from build123d import *

# Parameters (mm, degrees)
F1_DEPTH = 6.35
F3_DEPTH = 3.175


with BuildPart() as f1:
    # F0 (on Top) → F1 (new body)
    with BuildSketch(Plane.XY):
        with BuildLine():
            Line((44.45, 50.8), (-44.45, 50.8))
            ThreePointArc((-44.45, 50.8), (-48.940128, 48.940128), (-50.8, 44.45))
            Line((-50.8, 44.45), (-50.8, -44.45))
            ThreePointArc((-50.8, -44.45), (-48.940128, -48.940128), (-44.45, -50.8))
            Line((-44.45, -50.8), (44.45, -50.8))
            ThreePointArc((44.45, -50.8), (48.940128, -48.940128), (50.8, -44.45))
            Line((50.8, -44.45), (50.8, 44.45))
            ThreePointArc((50.8, 44.45), (48.940128, 48.940128), (44.45, 50.8))
        make_face()
    extrude(amount=F1_DEPTH)

    # F2 (on face) → F3 (cut)
    with BuildSketch(Plane.XY.offset(6.35)):
        Polygon((-2.234112, -19.045804), (-29.552355, -19.045804), (-29.552355, -21.484036), (-5.271634, -21.484036), (-5.271634, -27.478021), (-32.396957, -27.478021), (-32.396957, -31.338554), (-5.271634, -31.338554), (-5.271634, -37.027761), (-37.070233, -37.027761), (-37.070233, -24.125453), (-15.844628, 34.422915), (0, 34.422915), (15.844628, 34.422915), (37.070233, -24.125453), (37.070233, -37.027761), (5.271634, -37.027761), (5.271634, -31.338554), (32.396957, -31.338554), (32.396957, -27.478021), (5.271634, -27.478021), (5.271634, -21.484036), (29.552355, -21.484036), (29.552355, -19.045804), (2.234112, -19.045804), (2.234112, -40.488526), (41.246254, -40.488526), (41.246254, -24.237618), (17.566774, 37.974838), (0, 37.974838), (-17.566774, 37.974838), (-41.246254, -24.237618), (-41.246254, -40.488526), (-2.234112, -40.488526), align=None)
        with BuildLine():
            ThreePointArc((-9.515172, 23.211), (-17.458093, 10.48697), (-14.43387, -4.204695))
            ThreePointArc((-14.43387, -4.204695), (-2.520981, -10.7353), (10.401524, -6.543092))
            ThreePointArc((10.401524, -6.543092), (-4.451794, -8.46966), (-15.078945, 2.084788))
            ThreePointArc((-15.078945, 2.084788), (-12.326603, 15.929623), (0, 22.807829))
            ThreePointArc((0, 22.807829), (6.601318, 22.159177), (12.001306, 18.307129))
            ThreePointArc((12.001306, 18.307129), (14.956093, 7.863629), (9.017832, -1.221222))
            ThreePointArc((9.017832, -1.221222), (0.186781, -1.812212), (-5.294772, 5.136839))
            ThreePointArc((-5.294772, 5.136839), (-4.342036, 9.759367), (-0.376268, 12.318302))
            ThreePointArc((-0.376268, 12.318302), (-0.337375, 12.329109), (-0.301231, 12.347085))
            ThreePointArc((-0.301231, 12.347085), (3.122709, 12.777502), (5.674904, 10.454805))
            ThreePointArc((5.674904, 10.454805), (5.988125, 7.475454), (4.115821, 5.136839))
            ThreePointArc((4.115821, 5.136839), (1.688211, 5.89567), (0.35678, 8.062788))
            ThreePointArc((0.35678, 8.062788), (-0.732404, 6.827583), (-0.7692, 5.181162))
            ThreePointArc((-0.7692, 5.181162), (-0.749973, 5.13983), (-0.722364, 5.103558))
            ThreePointArc((-0.722364, 5.103558), (1.991164, 3.466413), (5.160289, 3.455573))
            ThreePointArc((5.160289, 3.455573), (8.487959, 7.340866), (7.337417, 12.325357))
            ThreePointArc((7.337417, 12.325357), (2.944683, 15.261206), (-2.33871, 15.228196))
            ThreePointArc((-2.33871, 15.228196), (-7.7104, 9.043988), (-7.555628, 0.854024))
            ThreePointArc((-7.555628, 0.854024), (-6.427229, -0.964786), (-4.758632, -2.305359))
            ThreePointArc((-4.758632, -2.305359), (5.051029, -4.221989), (14.110706, 0))
            ThreePointArc((14.110706, 0), (17.314869, 12.413903), (10.401524, 23.211))
            ThreePointArc((10.401524, 23.211), (0.443176, 25.849161), (-9.515172, 23.211))
        make_face()
    extrude(amount=-F3_DEPTH, mode=Mode.SUBTRACT)


solid = f1.part
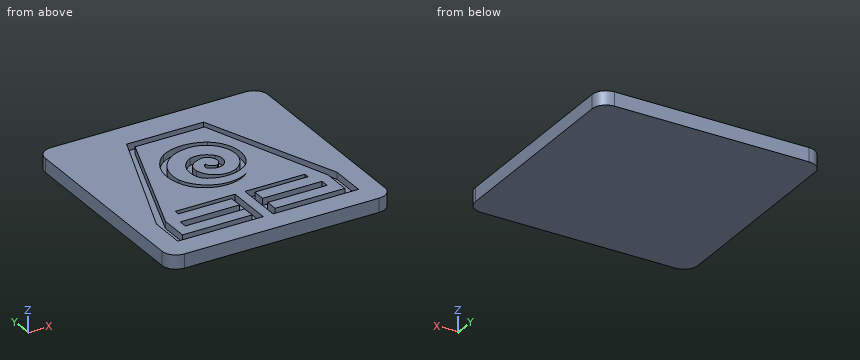
CAD build for the part. Positions are in the model's coordinates, mm. Round coordinates to 2 decimals unless told otherwise and drop trailing zeros. Write each loop counter-clockwise with the first axis right and the second up, starting at its lowest first coordinate (ties: lowest second). Pieces come first, ordered by that corner, then holes.
(1) Slice it at B-B, the plane y = -14. Write the cut outline in (x, z) (3 decimals).
(2) Drop a flat-ended pin along its axis: P1, Ø5, axis at x = 24, y = 31.5, coming from the -Z side. Give the stop position or say it passes through.
(3) Slice it at C-C, the plane z = 5.25. Count the separate pieces of the cut face and the enclosed holes in it, and give its area (3 significant figures).
(4) Probe line 1 along X through (y, z) = (21, 4); line 2 along X through (y, z) = (45, 1.25); line 3 along X through (y, z) = (-8, 6). List the from-to ranges inside material, lowest first.
(5) Slice it at D-D, the plane y = 27. Write the cut outline in (x, z) (3 decimals), and give its area (3 significant figures).
From the geometry:
1. outline: (-50.8, 0) - (50.8, 0) - (50.8, 6.35) - (37.35, 6.35) - (37.35, 3.175) - (33.399, 3.175) - (33.399, 6.35) - (-33.399, 6.35) - (-33.399, 3.175) - (-37.35, 3.175) - (-37.35, 6.35) - (-50.8, 6.35) - close
2. P1: stops at z = 0
3. separate pieces: 1
3. enclosed holes: 2
3. area: 8,540 mm2
4. line 1: x = -50.8 to -24.03, -20.71 to -12.06, -6.4 to 8.94, 13.04 to 20.71, 24.03 to 50.8
4. line 2: x = -50.78 to 50.78
4. line 3: x = -50.8 to -35.07, -31.22 to -10.32, -5.68 to 7.7, 8.49 to 31.22, 35.07 to 50.8
5. outline: (-50.8, 0) - (50.8, 0) - (50.8, 6.35) - (21.744, 6.35) - (21.744, 3.175) - (18.536, 3.175) - (18.536, 6.35) - (-18.536, 6.35) - (-18.536, 3.175) - (-21.744, 3.175) - (-21.744, 6.35) - (-50.8, 6.35) - close
5. area: 625 mm2
